Autodesk Fusion 360 part; units mm, degrees
sketch "Sketch1" plane through (0, 0, 0) normal (0, 1, 0) x (1, 0, 0)
  circle A0 centre (0, 0) radius 2.75
  circle A1 centre (0, 0) radius 5.75
  line L0 (-6, 0) -> (6, 0) construction
  dimension "d1" = 5.5
  dimension "d2" = 3
extrude "Extrude1" add sketch "Sketch1" against normal blind 10
sketch "Sketch2" plane through (0, 0, 0) normal (0, 1, 0) x (-1, 0, 0)
  circle A0 centre (0, 0) radius 2.75
  circle A1 centre (0, 0) radius 5.75
  line L0 (-6.5, 0) -> (6.5, 0) construction
  line L1 (0, -13.75) -> (0, 0) construction
  line L2 (-5.75, 0) -> (-5.75, -15) construction
  line L3 (5.75, 0) -> (5.75, -15) construction
  arc A2 (5.75, -10.7189) -> (0, -7.25) centre (0, -13.75) ccw
  arc A3 (0, -7.25) -> (-5.75, -10.7189) centre (0, -13.75) ccw
  line L4 (-5.75, -10.7189) -> (-5.75, 0)
  line L5 (5.75, -10.7189) -> (5.75, 0)
  dimension "d16" = 13.75
  dimension "d17" = 6.5
extrude "Extrude3" add sketch "Sketch2" against normal blind 2 contours A1 A2 A3 L4 L5
sketch "Sketch3" plane through (0, -2, 0) normal (0, -1, 0) x (1, 0, 0)
  arc A0 (5.75, -10.7189) -> (-5.75, -10.7189) centre (0, -13.75) ccw
  line L0 (5.75, -10.7189) -> (5.75, 0)
  arc A1 (-5.75, 0) -> (5.75, 0) centre (0, 0) ccw
  line L1 (-5.75, 0) -> (-5.75, -10.7189)
  arc A2 (5.75, -8.1879) -> (0, -5.75) centre (0, -13.75) ccw
  arc A3 (0, -5.75) -> (-5.75, -8.1879) centre (0, -13.75) ccw
  line L2 (-5.75, 0) -> (-5.75, -8.1879)
  line L3 (5.75, 0) -> (5.75, -8.1879)
  line L4 (-5.75, -8.1879) -> (0, -13.75) construction
  dimension "d24" = 8
extrude "Extrude4" add sketch "Sketch3" along normal blind 1.5 contours L0 A1 A2 L3 | A1 L1 A3 L2
sketch "Sketch5" plane through (0, -3.5, 0) normal (0, -1, 0) x (1, 0, 0)
  arc A0 (-5.75, 0) -> (0, -5.75) centre (0, 0) ccw
  line L0 (-5.75, 0) -> (-5.75, -8.1879)
  arc A1 (0, -5.75) -> (-5.75, -8.1879) centre (0, -13.75) ccw
  arc A2 (0, -7.25) -> (-5.75, -10.7189) centre (0, -13.75) ccw
  arc A3 (5.75, -10.7189) -> (0, -7.25) centre (0, -13.75) ccw
  line L1 (-5.75, -10.7189) -> (-5.75, 0)
  circle A4 centre (0, 0) radius 5.75
  line L2 (5.75, -10.7189) -> (5.75, 0)
  line L3 (0, -13.75) -> (0, 0)
  line L4 (0, -13.75) -> (-2.9897, -7.9784) construction
  dimension "d25" = 6.5
extrude "Extrude5" add sketch "Sketch5" along normal blind 2 contours A0 L0 A1 L1 A4 | A1 A2 L1 L3 | A3 A4 L2 L3
fillet "Fillet2" radius 1 2 edges at (5.75, -1, -10.7189) (5.75, -4.5, -10.7189)
fillet "Fillet4" radius 1 2 edges at (-5.75, -1, -10.7189) (-5.75, -4.5, -10.7189)
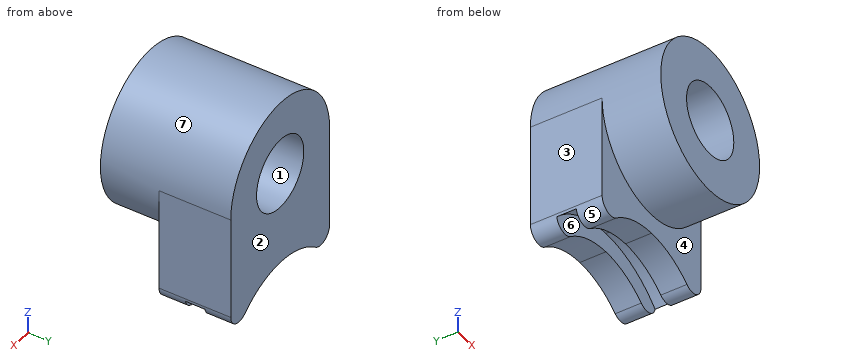
Read the model definition and answer for the solid it produces. Units are mm, in the model's axes. Face numbers are marked on the shaded views. A direction names the side the tool comes from. Give positions to 0.01 mm unless a question says otherwise; leave off trailing zeros. Order: outer loops, then holes, each group sorted by start corner. A loop starts at its lowest first (then second) coordinate and runs counter-clockwise, first axis right, second up. Notation, with made-up numbers: (-5.5, 7.25) -> (39.5, 7.25) arc R19 ccw to (39.5, 27.25) -> close; hole circle Ø2 at (55.5, 23). An arc over 180 degrees is marked (long way). One line per item, written item: value. Start each with the question number.
(1) For a pull along X with two mould halves and no side action, classify the marked faces 1, 2 and 3 as released by +X, released by -X, zero draft, split by the parting line, or undercut.
(2) A tool of negligible diameter and unlimited length cuts with its end or side. For the marked faces 4, 5, 6 and 7, from which of +Z, -Z, +X, -X, +Y, -Y can it reach the whole face along a straight path? Write none if from no direction.
(3) Flat-ended cylindrical pins translate along their axes: P1, Ø1, axis at x = 2.5, z = -6.5, coming from the -Y side; P2, Ø2, axis at x = 1, y = -7, coming from the -Z side. Find the tip coordinate at first contact, or state that the pin passes through.
(4) Straight lines are drawn through the part: L1, parallel to X at y = -4.75, z = 0; L2, parallel to Z at x = -1, y = -4.25. For each, find the intervals that lie inside material, in ascending order.
(5) The part is cut by section D-D (z = -6). Determine the outline of the cut face in (x, y), and give its area (3 significant figures).
(6) The part is cut by section A-A (y = -5). Determine the outline of the cut face in (x, z), and give its area (3 significant figures).
(7) The part is cut by section C-C (z = -2). Determine the outline of the cut face in (x, y), and give its area (3 significant figures).
(8) The part is cut by section B-B (x = -0.25). Determine the outline of the cut face in (y, z), and give its area (3 significant figures).
Taken from the geometry:
1. face 1: undercut
1. face 2: zero draft
1. face 3: released by -X
2. face 4: -Z, -Y
2. face 5: -Z, +Y, -Y
2. face 6: -Z
2. face 7: -Y
3. P1: y = -5.5
3. P2: z = -5.75
4. L1: -5.75 to -2.75, 2.75 to 5.75
4. L2: -7.33 to -2.56, 2.56 to 5.66
5. outline: (-5.75, -5.5) -> (5.75, -5.5) -> (5.75, 0) -> (-5.75, 0) -> close; hole (-1.98, -3.5) -> (1.98, -3.5) -> (1.98, -2) -> (-1.98, -2) -> close
5. area: 57.3 mm^2
6. outline: (-5.75, -7.95) arc R1 ccw to (-4.12, -8.72) arc R6.5 cw to (0, -7.25) arc R6.5 cw to (4.12, -8.72) arc R1 ccw to (5.75, -7.95) -> (5.75, 0) arc R5.75 ccw to (-5.75, 0) -> close; hole circle Ø5.5 at (0, 0)
6. area: 120 mm^2
7. outline: (-5.75, -5.5) -> (-5.39, -5.5) -> (-5.39, -10) -> (-1.89, -10) -> (-1.89, 0) -> (-5.75, 0) -> close; (1.89, -10) -> (5.39, -10) -> (5.39, -5.5) -> (5.75, -5.5) -> (5.75, 0) -> (1.89, 0) -> close
7. area: 74.0 mm^2
8. outline: (-10, -5.74) -> (-5.5, -5.74) -> (-5.5, -7.25) -> (-3.5, -7.25) -> (-3.5, -5.75) -> (-2, -5.75) -> (-2, -7.25) -> (0, -7.25) -> (0, -2.74) -> (-10, -2.74) -> close; (-10, 2.74) -> (0, 2.74) -> (0, 5.74) -> (-10, 5.74) -> close
8. area: 66.2 mm^2
